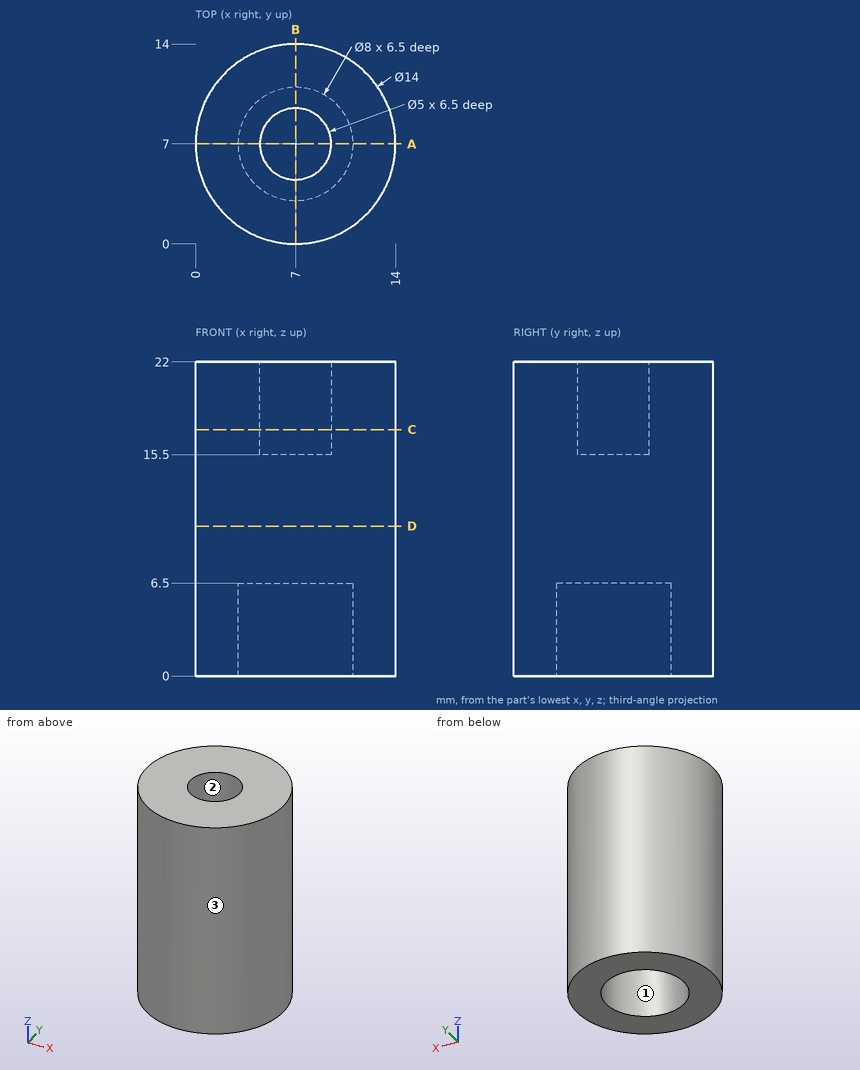
Input: dimensioned drawing with shaded views. Units: mm. Origin: part minimum x, y, z. A direction names the side the tool comes from. Coordinates: 2 decimals unless noted, no trailing zeros. Loops run counter-clockwise (first coordinate to the right, second up) from the corner with the lowest first, then second, coordinate; pieces in that order, holes last. Notation, with made-up numbers: M 19.25,34.5 L 24.25,34.5 A26 ccw 24.25,56.5 Z; hole C 36.5,-14.5 d6. An arc over 180 degrees is marked long. Put each result on its own line as item: value.
(1) Cut plane A-A on y = 7. Return the cut outline in (x, z), then the cut area to 4 significant figures.
Answer sheet:
outline: M 0,0 L 3,0 L 3,6.5 L 11,6.5 L 11,0 L 14,0 L 14,22 L 9.5,22 L 9.5,15.5 L 4.5,15.5 L 4.5,22 L 0,22 Z
area: 223.5 mm^2
(2) First-contact query: pin 1 (1.5 mm diameter, centred on x = 7.5, z = 13, fed in from -Y); pin 2 (4 mm diameter, centred on y = 4, z = 9, fed in from -X); pin 3 (3 mm diameter, centred on x = 11, z = 10, fed in from -Y); pin 4 (2 mm diameter, centred on x = 12, z = 17, fed in from +Y). Flat tips, straight axial feed; report the tip coordinate or a pass-through.
Answer sheet:
pin 1: stops at y = 0
pin 2: stops at x = 0.07
pin 3: stops at y = 0.46
pin 4: stops at y = 12.74
(3) Material intervals for probe 1 along Z at (x, y) = (7.5, 8.75); probe 2 along Y at (x, z) = (7, 4.75); probe 3 along Z at (x, y) = (9, 10.25), sorted ascending.
Answer sheet:
probe 1: z = 6.5 to 15.5
probe 2: y = 0 to 3, 11 to 14
probe 3: z = 6.5 to 22
(4) Access query for the marked faces 1, 2 and 3. Directions: +Z, -Z, +X, -X, +Y, -Y. A direction counts if a zero-diameter tool reaches every point of the face in a straight line with its end or side. Return the directions, or none.
Answer sheet:
face 1: -Z
face 2: +Z
face 3: +Z, -Z
(5) Cut plane D-D on z = 10.5. Return the cut outline in (x, y), then the cut area to 3 significant figures.
Answer sheet:
outline: C 7,7 d14
area: 154 mm^2
(6) Cut plane C-C on z = 17.25. Return the cut outline in (x, y), then the cut area to 3 significant figures.
Answer sheet:
outline: C 7,7 d14; hole C 7,7 d5
area: 134 mm^2
